Verification items for the finished model (mm, model axes). Face numbers are marked on the shaded views. A direction names the side the tool comes from. Round coordinates to 2 decimals unless told otherwise and drop trailing zeros. Write each loop counter-clockwise with the first axis right and the second up, starting at its lowest first coordinate (ties: lowest second). Pieces come first, ordered by that corner, then holes. Notation, with made-up numbers: (-16.75, 32.5) - (34.25, 32.5) arc R22 cw to (34.25, 63.5) - close; hole circle Ø9 at (10.25, 21.25). An arc over 180 degrees is marked (long way). Write each question's results on one line, items separated by ' | '.
```python
from build123d import *

# Parameters (mm, degrees)
F3_DEPTH = 3.81
F4_R     = 1.4478
F5_DEPTH = 25.4


with BuildPart() as f1:
    # F0 (on Right) → F1 (revolve)
    with BuildSketch(Plane.YZ):
        with BuildLine():
            Line((19.114999, 6.985), (0, 6.985))
            Line((0, 6.985), (0, 3.9751))
            Line((0, 3.9751), (28.8036, 3.9751))
            Line((28.8036, 3.9751), (28.8036, 11.303))
            Line((28.8036, 11.303), (24.4856, 11.303))
            Line((24.4856, 11.303), (24.4856, 12.7))
            Line((24.4856, 12.7), (20.6756, 12.7))
            Line((20.6756, 12.7), (20.6756, 8.770797))
            ThreePointArc((20.6756, 8.770797), (20.300805, 7.523529), (19.114999, 6.985))
        make_face()
    revolve(axis=Axis((0, 1.728549, 0), (0, 1, 0)))

    # F2 (on face) → F3 (join, through all)
    with BuildSketch(Plane.XZ.offset(-20.6756)):
        with BuildLine():
            Line((-12.7, 12.7), (-12.7, 0))
            ThreePointArc((-12.7, 0), (-8.980256, 8.980256), (0, 12.7))
            Line((0, 12.7), (-12.7, 12.7))
        make_face()
        with BuildLine():
            ThreePointArc((0, 12.7), (8.980256, 8.980256), (12.7, 0))
            Line((12.7, 0), (12.7, 12.7))
            Line((12.7, 12.7), (0, 12.7))
        make_face()
        with BuildLine():
            Line((0, -12.7), (12.7, -12.7))
            Line((12.7, -12.7), (12.7, 0))
            ThreePointArc((12.7, 0), (8.980256, -8.980256), (0, -12.7))
        make_face()
        with BuildLine():
            Line((-12.7, -12.7), (0, -12.7))
            ThreePointArc((0, -12.7), (-8.980256, -8.980256), (-12.7, 0))
            Line((-12.7, 0), (-12.7, -12.7))
        make_face()
    extrude(amount=-F3_DEPTH)

    # F4 (on face) → F5 (cut)
    with BuildSketch(Plane.XZ.offset(-20.6756)):
        with Locations((10.0584, -10.0584)):
            Circle(F4_R)
        with Locations((10.0584, 10.0584)):
            Circle(F4_R)
        with Locations((-10.0584, -10.0584)):
            Circle(F4_R)
        with Locations((-10.0584, 10.0584)):
            Circle(F4_R)
    extrude(amount=-F5_DEPTH, mode=Mode.SUBTRACT)


solid = f1.part
```
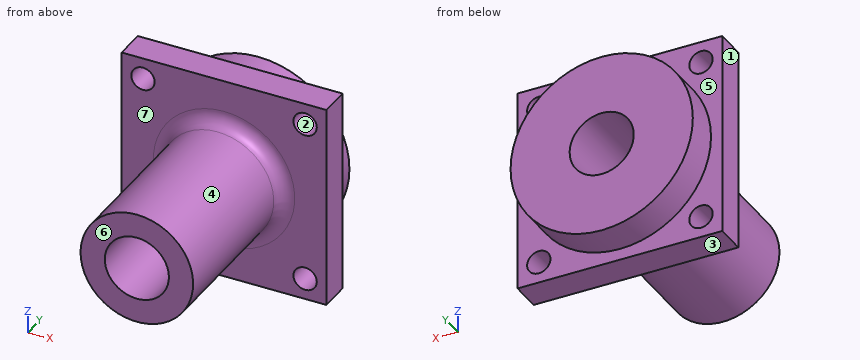
(1) Go/stop test with flat-tipped pins: pin 1 Ø7 at (x, z) = (0, 0) entering from -Y; pin 2 Ø6 at (x, y) = (1.5, 25) entering from +Z; pin 3 Ø1.5 at (x, z) = (2, 8) entering from -Y; pin 4 Ø8 at (y, z) = (8.5, -4.5) entering from +X. Record where each tip stops, or that it passes through.
Answer:
pin 1: through | pin 2: z = 12.7 | pin 3: y = 20.28 | pin 4: x = 6.97
(2) Mould release check, pull along Z, two halves, no side actions. Record for the marked faces 1, 2, 3 and 4: released by +Z, released by -Z, zero draft, split by the parting line, or undercut.
Answer:
face 1: zero draft | face 2: undercut | face 3: released by -Z | face 4: split by the parting line
(3) Section check B-B (x = 0). Record the cut outline in (y, z) (3 decimals).
Answer:
outline: (0, -6.985) - (19.115, -6.985) arc R1.575 cw to (20.676, -8.771) - (20.676, -12.7) - (24.486, -12.7) - (24.486, -11.303) - (28.804, -11.303) - (28.804, -3.975) - (0, -3.975) - close; (0, 3.975) - (28.804, 3.975) - (28.804, 11.303) - (24.486, 11.303) - (24.486, 12.7) - (20.676, 12.7) - (20.676, 8.771) arc R1.575 cw to (19.115, 6.985) - (0, 6.985) - close
(4) Thickness scan on L1, parallel to Y at x = -8.5, z = -9.75; L2, parallel to Z at x = 0.5, y = 7.5; L3, parallel to Z at x = 0.5, y = 26.5. Record the ranges inside material, lowest first.
Answer:
L1: 20.68 to 24.49 | L2: -6.97 to -3.94, 3.94 to 6.97 | L3: -11.29 to -3.94, 3.94 to 11.29
(5) Section check C-C (y = 7.25). Record the cut outline in (x, z) (3 decimals), plus the area to 3 significant figures.
Answer:
outline: circle Ø13.97 at (0, 0); hole circle Ø7.95 at (0, 0) | area: 104 mm2
(6) Section check A-A (z = 0). Record the cut outline in (x, y) (3 decimals), plus the area to 3 significant figures.
Answer:
outline: (-12.7, 20.676) - (-8.771, 20.676) arc R1.575 cw to (-6.985, 19.115) - (-6.985, 0) - (-3.975, 0) - (-3.975, 28.804) - (-11.303, 28.804) - (-11.303, 24.486) - (-12.7, 24.486) - close; (3.975, 0) - (6.985, 0) - (6.985, 19.115) arc R1.575 cw to (8.771, 20.676) - (12.7, 20.676) - (12.7, 24.486) - (11.303, 24.486) - (11.303, 28.804) - (3.975, 28.804) - close | area: 255 mm2
(7) Set-up check for the marked faces 5, 6 and 7: record each of +Z, -Z, +X, -X, +Y, -Y from which the full face is reachable in a straight line by a thin tool's end or side.
Answer:
face 5: +Y | face 6: +Z, -Z, +X, -X, -Y | face 7: -Y
